Autodesk Inventor part; units mm, degrees
ref_plane "YZ Plane" through (0, 0, 0) normal (1, 0, 0) x (0, 1, 0)
ref_plane "XZ Plane" through (0, 0, 0) normal (0, 1, 0) x (-1, 0, 0)
ref_plane "XY Plane" through (0, 0, 0) normal (0, 0, 1) x (1, 0, 0)
sketch "Sketch1" plane through (0, 0, 0) normal (0, 1, 0) x (-1, 0, 0)
  line L0 (47.6597, 73.3148) -> (47.6597, 78.3148)
  line L1 (97.6593, 78.3148) -> (97.6593, 72.863)
  line L2 (-82.3403, 73.3148) -> (-82.3403, 78.3148)
  line L3 (-32.3403, 78.3148) -> (-32.3403, 73.3148)
  line L4 (117.6597, 72.863) -> (97.6593, 72.863)
  line L5 (47.6597, 73.3148) -> (-32.3403, 73.3148)
  line L6 (-82.3403, 73.3148) -> (-107.3403, 73.3148)
  line L7 (-20.3403, 63.3147) -> (-44.3403, 63.3147)
  line L8 (-47.3403, 60.3147) -> (-47.3403, 41.3147)
  line L9 (-44.3403, 38.3147) -> (-20.3403, 38.3147)
  line L10 (-17.3403, 41.3147) -> (-17.3403, 60.3147)
  line L11 (29.6597, 63.3147) -> (15.6597, 63.3147)
  line L12 (12.6597, 60.3147) -> (12.6597, 46.3147)
  line L13 (15.6597, 43.3147) -> (29.6597, 43.3147)
  line L14 (32.6597, 46.3147) -> (32.6597, 60.3147)
  arc A0 (29.6597, 43.3147) -> (32.6597, 46.3147) centre (29.6597, 46.3147) ccw
  arc A1 (32.6597, 60.3147) -> (29.6597, 63.3147) centre (29.6597, 60.3147) ccw
  arc A2 (15.6597, 63.3147) -> (12.6597, 60.3147) centre (15.6597, 60.3147) ccw
  arc A3 (12.6597, 46.3147) -> (15.6597, 43.3147) centre (15.6597, 46.3147) ccw
  arc A4 (-20.3403, 38.3147) -> (-17.3403, 41.3147) centre (-20.3403, 41.3147) ccw
  arc A5 (-47.3403, 41.3147) -> (-44.3403, 38.3147) centre (-44.3403, 41.3147) ccw
  arc A6 (-44.3403, 63.3147) -> (-47.3403, 60.3147) centre (-44.3403, 60.3147) ccw
  arc A7 (-17.3403, 60.3147) -> (-20.3403, 63.3147) centre (-20.3403, 60.3147) ccw
  line L15 (97.6597, -36.6853) -> (117.6597, -36.6853)
  line L16 (-107.3403, -36.6853) -> (-82.3403, -36.6853)
  line L17 (-32.3403, -36.6853) -> (47.6597, -36.6853)
  line L18 (-107.3403, 0.8147) -> (-107.3403, -36.6853)
  line L19 (-107.3403, 0.8147) -> (-102.3403, 0.8147)
  line L20 (-102.3403, 0.8147) -> (-102.3403, 35.8147)
  line L21 (-102.3403, 35.8147) -> (-107.3403, 35.8147)
  line L22 (-107.3403, 35.8147) -> (-107.3403, 73.3148)
  line L23 (117.6597, -36.6853) -> (122.6597, -36.6853)
  line L24 (122.6597, -36.6853) -> (122.6597, 0.8147)
  line L25 (122.6597, 0.8147) -> (117.6597, 0.8147)
  line L26 (117.6597, 0.8147) -> (117.6597, 35.8147)
  line L27 (122.6902, 35.8147) -> (122.6902, 72.863)
  line L28 (122.6902, 72.863) -> (117.6597, 72.863)
  line L29 (122.6902, 35.8147) -> (117.6597, 35.8147)
  line L30 (97.6597, -36.6853) -> (-82.3403, -36.6853)
  line L31 (-32.3403, 73.3148) -> (-32.3403, 78.3148)
  line L32 (-32.3403, 78.3148) -> (-82.3403, 78.3148)
  line L33 (47.6597, 78.3148) -> (97.6593, 78.3148)
  point P0 (-17.3403, 63.3147)
  point P1 (-47.3403, 63.3147)
  point P2 (-47.3403, 38.3147)
  point P3 (32.6597, 63.3147)
  point P4 (12.6597, 63.3147)
  point P5 (12.6597, 43.3147)
  dimension "d4" = 80
  dimension "d19" = 30
  dimension "d20" = 25
  dimension "d28" = 20
  dimension "d29" = 20
  dimension "d30" = 30
  dimension "d31" = 3
  dimension "d41" = 5
  dimension "d53" = 5
extrude "Extrusion3" add sketch "Sketch1" along normal blind 5
properties part number "Part Sisi 3"
For this review, take the finished solid that the model builds, in its own axes (mm). A direction names the side the tool comes from. Coordinates: 2 decimals unless noted, no trailing zeros. Order: outer loops, then holes, each group sorted by start corner. A loop starts at its lowest first (then second) coordinate and runs counter-clockwise, first axis right, second up. Notation, with made-up numbers: (18, 79.25) -> (39, 79.25) arc R17 cw to (39, 98.25) -> close; hole circle Ø2 at (49, -21). An arc over 180 degrees is marked (long way). Use CSV: the item, a comma, the result in double quotes. Start each with the question number.
Item 1: Wall thickness on probe 1 along X at (y, z) = (2.2, 55); probe 2 along Z at (x, y) = (43.5, 1.2); probe 3 along Z at (x, y) = (22, 3.25): over which ranges is each line inside the solid? List them lowest first.
Item 2: Draft analysis for pull direction X (two halves, no side actions). For faces 4 (the face through (105, 2, 35.815)), 5 (the face through (-97.659, 2, 76)), 6 (the face through (-23, 2, 43.315)), 7 (the face through (102.34, 2, 18)), state which applies: pulls with the +X half, pulls with the -X half, needs draft (parallel to the pull), parting line crosses it, or undercut.
Item 3: We need section C-C, the plane x = 8.5. Give the boundary of the cut face in (y, z), then the cut area to 3 significant figures.
Item 4: We need section B-B, the plane y = 1.3. Give the number of separate pieces and of enclosed holes in the cut face, then the cut area to 3 significant figures.
Item 5: We need section D-D, the plane z = 30. Give the boundary of the cut face in (x, y), then the cut area to 3 significant figures.
Item 6: We need section A-A, the plane z = 51. Give the boundary of the cut face in (x, y), then the cut area to 3 significant figures.
Item 7: Insertion check: pin 1 (2.5 mm diameter, centred on x = -120.5, y = 2, fed in from +Z); pin 2 (1 mm diameter, centred on y = 4.5, z = -1.5, fed in from -X); pin 3 (1.5 mm diameter, centred on y = 2, z = 76.5, fed in from +X). Each pin has a flat end and moves straight along its axis. Give the tip position at first contact, or say it passes through.
Item 8: For faces 1 (the face through (-23, 2, 63.315)), 2 (the face through (105, 2, 0.815)), 3 (the face through (-47.66, 2, 76)), list the 3-axis set-ups (+Z, -Z, +X, -X, +Y, -Y) from which the entire face can be reached by the end or side of a thin tool; tool diameter is ignored.
Derived:
1,probe 1,"x = -122.69 to -32.66, -12.66 to 17.34, 47.34 to 107.34"
1,probe 2,"z = -36.69 to 38.31, 63.31 to 78.31"
1,probe 3,"z = -36.69 to 38.31, 63.31 to 73.31"
2,face 4,"needs draft"
2,face 5,"pulls with the -X half"
2,face 6,"undercut"
2,face 7,"pulls with the +X half"
3,outline,"(0, -36.69) -> (5, -36.69) -> (5, 73.31) -> (0, 73.31) -> close"
3,area,"550 mm^2"
4,separate pieces,"1"
4,enclosed holes,"2"
4,area,"24,300 mm^2"
5,outline,"(-117.66, 0) -> (102.34, 0) -> (102.34, 5) -> (-117.66, 5) -> close"
5,area,"1,100 mm^2"
6,outline,"(-122.69, 0) -> (-32.66, 0) -> (-32.66, 5) -> (-122.69, 5) -> close; (-12.66, 0) -> (17.34, 0) -> (17.34, 5) -> (-12.66, 5) -> close; (47.34, 0) -> (107.34, 0) -> (107.34, 5) -> (47.34, 5) -> close"
6,area,"900 mm^2"
7,pin 1,"stops at z = 72.86"
7,pin 2,"stops at x = -122.66"
7,pin 3,"stops at x = 82.34"
8,face 1,"+Y, -Y"
8,face 2,"+X, +Y, -Y"
8,face 3,"+Z, +Y, -Y"
